For this review, use the dimensioned drawing (mm, ordinates from the lowest corner) and the shaded views. A direction names the side the tool comes from. Coordinates: 2 decimals unless noted, no trailing zeros. Order: outer loops, then holes, each group sorted by start corner. A loop starts at its lowest first (then second) coordinate and runs counter-clockwise, first axis right, second up. Notation, with made-up numbers: M -32,57 L 21,57 A24 ccw 21,83 Z; hole C 55.25,61 d3. An arc over 180 degrees is marked long. Answer as CSV lines item,"result". Start each with the question number.
Q1. Consider section C-C on y = 2.25. Write out the cut boundary in (x, z), and give its area (3 significant figures).
Q2. Machinability: for the marked faces 1, 2 and 3, which of the approach directions +Z, -Z, +X, -X, +Y, -Y give a long, thin tool a straight path to every point of the face, cutting with its end or side? Answer none if there is none.
Q3. Wall thickness on L1, parallel to X at y = 1.5, z = 2.5; L2, parallel to X at y = 0.85, z = 14.5; L3, parallel to Y at x = 41, z = 4.5: over which ranges is each line inside the solid? List them lowest first. Write a range as [from, to].
Q4. For P1, Ø1.1, axis at y = 0.5, z = 6.5, coming from the +X side; P2, Ø1, axis at y = 2.5, z = 9, coming from the +X side; P3, Ø4, axis at x = 1.5, z = 14, coming from the +Y side, all flat-tipped, find the tip position at first contact; note any pin that passes through.
Q5. Consider section A-A on z = 16.5. Write out the cut boundary in (x, y), and give its area (3 significant figures).
Q6. Consider section B-B on z = 14. Write out the cut boundary in (x, y).
Q7. Consider section D-D on x = 3. Write out the cut boundary in (y, z), and give its area (3 significant figures).
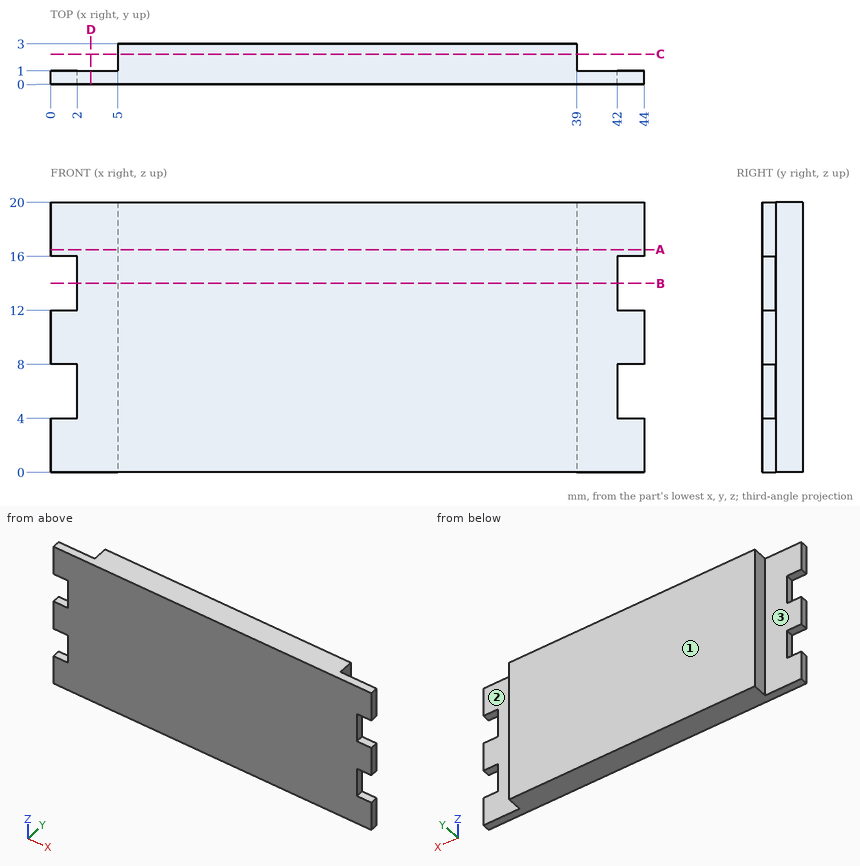
Evaluation:
1,outline,"M 5,0 L 39,0 L 39,20 L 5,20 Z"
1,area,"680 mm²"
2,face 1,"+Z, -Z, +X, -X, +Y"
2,face 2,"+Z, -Z, +X, +Y"
2,face 3,"+Z, -Z, -X, +Y"
3,L1,"x = [5, 39]"
3,L2,"x = [2, 42]"
3,L3,"y = [0, 1]"
4,P1,"stops at x = 42"
4,P2,"stops at x = 39"
4,P3,"stops at y = 1"
5,outline,"M 0,0 L 44,0 L 44,1 L 39,1 L 39,3 L 5,3 L 5,1 L 0,1 Z"
5,area,"112 mm²"
6,outline,"M 2,0 L 42,0 L 42,1 L 39,1 L 39,3 L 5,3 L 5,1 L 2,1 Z"
7,outline,"M 0,0 L 1,0 L 1,20 L 0,20 Z"
7,area,"20.0 mm²"
